```python
from build123d import *

# Parameters (mm, degrees)
SKETCH1_R             = 3
STEERING_COLUMN_DEPTH = 30
LEFT_HANDLE_BAR_DEPTH = 5


with BuildPart() as part:
    # Sketch1 → Steering Column (new body)
    with BuildSketch(Plane(origin=(0, 0, 0), x_dir=(1, 0, 0), z_dir=(0, 1, 0))):
        with Locations(Location((0, 0, 0), (0, 0, 270))):
            Circle(SKETCH1_R)
    extrude(amount=STEERING_COLUMN_DEPTH)

    # Sketch2 → Left Handle Bar (add)
    with BuildSketch(Plane(origin=(0, 30, 0), x_dir=(1, 0, 0), z_dir=(0, 1, 0))):
        Polygon((2.598076211, 1.5), (-14.300966168, 30.77), (-31.033016975, 30.77), (-31.033016975, 24.77), (-17.765067783, 24.77), (-2.598076211, -1.5), align=None)
    left_handle_bar = extrude(amount=-LEFT_HANDLE_BAR_DEPTH)

    # Mirror1: Left Handle Bar across plane
    add(left_handle_bar.mirror(Plane.XY))


solid = part.part
```
CAD build for the part. Positions are in the model's coordinates, mm. A direction names the side the tool comes from. Round coordinates to 2 decimals unless told otherwise and drop trailing zeros. Loops run counter-clockwise (first coordinate to the right, second up) from the corner with the lowest first, then second, coordinate; pieces in that order, holes last. Notation, with made-up numbers: M -0.5,42 L 52.5,42 A31 cw 52.5,79 Z; hole C 64,28 d2. An arc over 180 degrees is marked long. Return JSON: item names as keys, results as strings. Group by question number.
(1) Wall check: probe 1 along Y at (x, z) = (-26.5, -27); probe 2 along Z at (x, y) = (-6.5, 25.5); probe 3 along X at (y, z) = (28.5, 4.5). Give the ranges that are in metal, low to high. Write a range as [from, to].
(2) Mould opens along Z. For faces 1 (the flat face through (0, 0, 0)), 2 (the flat face through (-23, 28, -30.77)), 3 (the flat face through (-24, 28, 24.77)) say: +Z half, -Z half, draft (parallel to the pull), parting line (faces both ways), or undercut.
(3) Tool access for faces 4 (the cylindrical face through (3, 15, 0)), 5 (the flat face through (-10.715, 27.535, 12.558)), 6 (the flat face through (-5.733, 27.535, 15.93)): list every direction of +Z, -Z, +X, -X, +Y, -Y with a clear straight run to the whole face (end or side of a thin tool).
(4) Drop flat-ended pins along their axis: P1, Ø1.5, axis at x = -8.5, z = -21, coming from the -Y side; P2, Ø6, axis at y = 25.5, z = -21, coming from the -X side. Give the stop position or say it passes through.
(5) Saw through at C-C, the plane x = 0. List the corners of the cut face in (y, z), and give its area (3 significant figures).
(6) Saw through at D-D, the plane x = -12.5. List the corners of the cut face in (y, z).
(7) Saw through at B-B, the plane y = 26.5. List the corners of the cut face in (x, z), and give its area (3 significant figures).
(8) Saw through at A-A, the plane x = -21. List the corners of the cut face in (y, z), and give its area (3 significant figures).
Answer list:
{
 "1": {"probe 1": "[25, 30]", "probe 2": "[-17.26, -5.26], [5.26, 17.26]", "probe 3": "[-6.06, 0.87]"},
 "2": {"face 1": "draft", "face 2": "-Z half", "face 3": "undercut"},
 "3": {"face 4": "-Y", "face 5": "-X, +Y, -Y", "face 6": "+Z, +X, +Y, -Y"},
 "4": {"P1": "y = 25", "P2": "x = -17.32"},
 "5": {"outline": "M 0,-3 L 25,-3 L 25,-6 L 30,-6 L 30,6 L 25,6 L 25,3 L 0,3 Z", "area": "210 mm2"},
 "6": {"outline": "M 25,-27.65 L 30,-27.65 L 30,-15.65 L 25,-15.65 Z; M 25,15.65 L 30,15.65 L 30,27.65 L 25,27.65 Z"},
 "7": {"outline": "M -31.03,-30.77 L -14.3,-30.77 L 2.6,-1.5 A3 ccw 2.6,1.5 L -14.3,30.77 L -31.03,30.77 L -31.03,24.77 L -17.77,24.77 L -3.46,0 L -17.77,-24.77 L -31.03,-24.77 Z", "area": "564 mm2"},
 "8": {"outline": "M 25,-30.77 L 30,-30.77 L 30,-24.77 L 25,-24.77 Z; M 25,24.77 L 30,24.77 L 30,30.77 L 25,30.77 Z", "area": "60.0 mm2"}
}
